```python
from build123d import *

# Parameters (mm, degrees)
F0_R     = 27.5
F0_R_2   = 1
F0_R_3   = 21.1
F1_DEPTH = 10
F3_DEPTH = 10
F5_W     = 4
F5_H     = 4
F5_R     = 1
F6_DEPTH = 5


# Not quite as in the source:
# - a fillet or chamfer that OpenCascade refuses, or shapes differently, is made with other operations: its cross-section is extruded or revolved along the edge and cut away or added


with BuildPart() as f1:
    # F0 (on Top) → F1 (new body)
    with BuildSketch(Plane.XY):
        Circle(F0_R)
        with Locations((-17.1119841047, -17.1119841047)):
            Circle(F0_R_2, mode=Mode.SUBTRACT)
        with Locations((0, -24.2)):
            Circle(F0_R_2, mode=Mode.SUBTRACT)
        with Locations((17.1119841047, -17.1119841047)):
            Circle(F0_R_2, mode=Mode.SUBTRACT)
        with Locations((-24.2, 0)):
            Circle(F0_R_2, mode=Mode.SUBTRACT)
        with Locations((-17.1119841047, 17.1119841047)):
            Circle(F0_R_2, mode=Mode.SUBTRACT)
        Circle(F0_R_3, mode=Mode.SUBTRACT)
        with Locations((24.2, 0)):
            Circle(F0_R_2, mode=Mode.SUBTRACT)
        with Locations((0, 24.2)):
            Circle(F0_R_2, mode=Mode.SUBTRACT)
        with Locations((17.1119841047, 17.1119841047)):
            Circle(F0_R_2, mode=Mode.SUBTRACT)
        Circle(F0_R_3)
        with BuildLine():
            ThreePointArc((1.4936867141, 1.33), (0, -2), (-1.4936867141, 1.33))
            Line((-1.4936867141, 1.33), (1.4936867141, 1.33))
        make_face(mode=Mode.SUBTRACT)
    extrude(amount=F1_DEPTH)

    # F2: chamfer of 5 on 1 edges, made by hand

    # F2_s1 → F2_t2 (revolve, cut)
    with BuildSketch(Plane.XZ):
        Polygon((27.5, 5), (22.5, 10), (27.5, 10), align=None)
    revolve(axis=Axis((0, 0, 10), (0, 0, 1)), mode=Mode.SUBTRACT)

    # F0 (on Top) → F3 (cut)
    with BuildSketch(Plane.XY):
        with BuildLine():
            Line((1.4936867141, 1.33), (-1.4936867141, 1.33))
            ThreePointArc((-1.4936867141, 1.33), (0, -2), (1.4936867141, 1.33))
        make_face()
    extrude(amount=F3_DEPTH, mode=Mode.SUBTRACT)

    # F5 (on offset) → F6 (cut)
    with BuildSketch(Plane.XY.offset(5)):
        with Locations((0, 24.2)):
            Rectangle(F5_W, F5_H)
        with Locations((0, 24.2)):
            Circle(F5_R, mode=Mode.SUBTRACT)
        with Locations((0, 24.2)):
            Circle(F5_R)
        Polygon((-14.28355698, 17.1119841047), (-17.1119841047, 19.9404112295), (-19.9404112295, 17.1119841047), (-17.1119841047, 14.28355698), align=None)
        Polygon((17.1119841047, 14.28355698), (19.9404112295, 17.1119841047), (17.1119841047, 19.9404112295), (14.28355698, 17.1119841047), align=None)
        with Locations((-24.2, 0)):
            Rectangle(F5_W, F5_H)
        Polygon((-17.1119841047, -14.28355698), (-19.9404112295, -17.1119841047), (-17.1119841047, -19.9404112295), (-14.28355698, -17.1119841047), align=None)
        with Locations((0, -24.2)):
            Rectangle(F5_W, F5_H)
        Polygon((14.28355698, -17.1119841047), (17.1119841047, -19.9404112295), (19.9404112295, -17.1119841047), (17.1119841047, -14.28355698), align=None)
        with Locations((24.2, 0)):
            Rectangle(F5_W, F5_H)
    extrude(amount=F6_DEPTH, mode=Mode.SUBTRACT)


solid = f1.part
```
Part model, mm, in its own coordinate system. A direction names the side the tool comes from. Round coordinates to 2 decimals unless told otherwise and drop trailing zeros. Loops run counter-clockwise (first coordinate to the right, second up) from the corner with the lowest first, then second, coordinate; pieces in that order, holes last.
Item 1: Mould opens along X. For faces 3 (the face through (-5.961, -26.846, 2.465)), 4 (the face through (0, -6, 0)), 5 (the face through (-25, 1, 5)) say: +X half, -X half, draft (parallel to the pull), parting line (faces both ways), or undercut.
Item 2: Drop flat-ended pins along their axis: P1, Ø3, axis at y = 2.5, z = 5.5, coming from the +X side; P2, Ø3, axis at y = 1, z = 7.5, coming from the -X side; P3, Ø0.6, axis at y = 0.5, z = 6, coming from the +X side. Give the stop position or say it passes through.
Item 3: 3-axis set-ups, long thin cutter, end or side, ignore diameter. For faces 1 (the face through (18.066, -16.812, 2.465)), 2 (the face through (18.546, 18.506, 5.641)): which of +Z, -Z, +X, -X, +Y, -Y reach the whole face in a straight line?
Item 4: Drill centre lines: line 1 (Y direction, x = -16, z = 5.25); line 2 (X direction, y = -24.2, z = 2.8). Where is each one in solid material? Low to high.
Item 5: Cut at B-B, the plane x = 0. Give the cut face in (y, z).
Item 6: Cut at A-A, the plane y = 0. Give the cut face in (x, z).
A:
1. face 3: parting line
1. face 4: draft
1. face 5: undercut
2. P1: stops at x = 27.48
2. P2: stops at x = -26.48
2. P3: stops at x = 26.8
3. face 1: +Z, -Z
3. face 2: +Z
4. line 1: y = -22.06 to -18.83, -15.4 to 15.4, 18.83 to 22.06
4. line 2: x = -13.06 to -1, 1 to 13.06
5. outline: (-27.5, 0) - (-25.2, 0) - (-25.2, 5) - (-26.2, 5) - (-26.2, 6.3) - (-27.5, 5) - close; (-23.2, 0) - (-2, 0) - (-2, 10) - (-22.2, 10) - (-22.2, 5) - (-23.2, 5) - close; (1.33, 0) - (23.2, 0) - (23.2, 5) - (22.2, 5) - (22.2, 10) - (1.33, 10) - close; (25.2, 0) - (27.5, 0) - (27.5, 5) - (26.2, 6.3) - (26.2, 5) - (25.2, 5) - close
6. outline: (-27.5, 0) - (-25.2, 0) - (-25.2, 5) - (-26.2, 5) - (-26.2, 6.3) - (-27.5, 5) - close; (-23.2, 0) - (-2, 0) - (-2, 10) - (-22.2, 10) - (-22.2, 5) - (-23.2, 5) - close; (2, 0) - (23.2, 0) - (23.2, 5) - (22.2, 5) - (22.2, 10) - (2, 10) - close; (25.2, 0) - (27.5, 0) - (27.5, 5) - (26.2, 6.3) - (26.2, 5) - (25.2, 5) - close
